The listing builds one solid part. Answer for the finished solid, in the listing's coordinates (mm). Face numbers are marked on the shaded views. A direction names the side the tool comes from. Round coordinates to 2 decimals unless told otherwise and drop trailing zeros. Loops run counter-clockwise (first coordinate to the right, second up) from the corner with the lowest first, then second, coordinate; pieces in that order, holes last. Notation, with made-up numbers: (88, 53.25) - (108, 53.25) arc R27 ccw to (108, 71.25) - close; hole circle Ø8 at (-5, -18). An arc over 180 degrees is marked (long way). Write item = value, one per line. Start each with the question number.
1) Given pin 1 Ø15 at (y, z) = (-5.5, 38) entering from -X; pin 2 Ø5 at (x, z) = (19.5, 20.5) entering from -Y; pin 3 Ø12 at (x, y) = (28.5, 0.5) entering from +Z; pin 4 Ø15 at (y, z) = (-5, 27.5) entering from +X, each flat-ended and moving along its own axis, determine where each tip first touches the part or whether it passes through.
2) Section B-B, the plane y = 17 is taken. Determine the outline of the cut face in (x, z).
3) Section C-C, the plane x = 20.5 is taken. Determine the outline of the cut face in (y, z), and give its area (3 significant figures).
4) Section D-D, the plane x = -31 is taken. Determine the outline of the cut face in (y, z).
5) A tool of negligible diameter and unlimited length cuts with its end or side. For the marked faces 4, 5, 6 and 7, from which of +Z, -Z, +X, -X, +Y, -Y can it reach the whole face along a straight path? Write none if from no direction.
6) Section A-A, the plane z = 26 is taken. Determine the outline of the cut face in (x, y).
7) For a pull along X with two mould halves and no side action, classify the marked faces 1, 2 and 3 as released by +X, released by -X, zero draft, split by the parting line, or undercut.
8) Straight lines are drawn through the part: line 1 along Y through (x, z) = (30, 6); line 2 along X through (y, z) = (17, 7); line 3 along X through (y, z) = (2.5, 22.5). For each, find the intervals that lie inside material, in ascending order.
from build123d import *

# Parameters (mm, degrees)
SKETCH_1_W          = 80
SKETCH_1_H          = 50
EXTRUDE_1_DEPTH     = 10
EXTRUDE_2_DEPTH     = 10
SKETCH_3_R          = 6
CUT_EXTRUDE_1_DEPTH = 86.732140997
SKETCH_4_R          = 4.5
CUT_EXTRUDE_2_DEPTH = 69.738635424


with BuildPart() as part:
    # 草图1 → 凸台-拉伸1 (new body)
    with BuildSketch(Plane.XY):
        Rectangle(SKETCH_1_W, SKETCH_1_H)
    extrude(amount=EXTRUDE_1_DEPTH)

    # 草图2 → 凸台-拉伸2 (add)
    with BuildSketch(Plane(origin=(15, 0, 0), x_dir=(0, 0, -1), z_dir=(1, 0, 0))):
        with BuildLine():
            Line((-9.5, -15), (-35, -15))
            ThreePointArc((-35, -15), (-50, 0), (-35, 15))
            Line((-35, 15), (-9.5, 15))
            Line((-9.5, 15), (-9.5, -15))
        make_face()
    extrude_2 = extrude(amount=EXTRUDE_2_DEPTH)

    # 镜向1: 凸台-拉伸2 across plane
    add(extrude_2.mirror(Plane(origin=(0, 0, 0), x_dir=(0, 0, 1), z_dir=(1, 0, 0))))

    # 草图3 → 切除-拉伸1 (cut, through all)
    with BuildSketch(Plane(origin=(-25, 0, 0), x_dir=(0, 0, -1), z_dir=(1, 0, 0))):
        with Locations((-35, 0)):
            Circle(SKETCH_3_R)
    extrude(amount=CUT_EXTRUDE_1_DEPTH, mode=Mode.SUBTRACT)

    # 草图4 → 切除-拉伸2 (cut, through all)
    with BuildSketch(Plane.XY):
        with Locations((30, 17)):
            Circle(SKETCH_4_R)
        with Locations((30, -17)):
            Circle(SKETCH_4_R)
        with Locations((-30, 17)):
            Circle(SKETCH_4_R)
        with Locations((-30, -17)):
            Circle(SKETCH_4_R)
    extrude(amount=CUT_EXTRUDE_2_DEPTH, mode=Mode.SUBTRACT)


solid = part.part
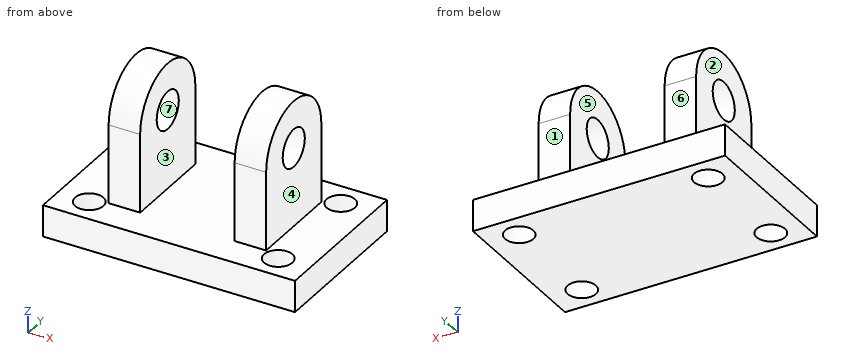
Geometry check:
q1.pin_1 = -25
q1.pin_2 = -15
q1.pin_3 = 50
q1.pin_4 = 25
q2.outline = (-40, 0) - (-34.5, 0) - (-34.5, 10) - (-40, 10) - close; (-25.5, 0) - (25.5, 0) - (25.5, 10) - (-25.5, 10) - close; (34.5, 0) - (40, 0) - (40, 10) - (34.5, 10) - close
q3.outline = (-25, 0) - (25, 0) - (25, 10) - (15, 10) - (15, 35) arc R15 ccw to (-15, 35) - (-15, 10) - (-25, 10) - close; hole circle Ø12 at (0, 35)
q3.area = 1,490 mm2
q4.outline = (-25, 0) - (-21.39, 0) - (-21.39, 10) - (-25, 10) - close; (-12.61, 0) - (12.61, 0) - (12.61, 10) - (-12.61, 10) - close; (21.39, 0) - (25, 0) - (25, 10) - (21.39, 10) - close
q5.face_4 = +Z, +X, +Y, -Y
q5.face_5 = +Z, +Y, -Y
q5.face_6 = +Z, +X, -X, +Y
q5.face_7 = +X, -X
q6.outline = (-25, -15) - (-15, -15) - (-15, 15) - (-25, 15) - close; (15, -15) - (25, -15) - (25, 15) - (15, 15) - close
q7.face_1 = zero draft
q7.face_2 = released by -X
q7.face_3 = undercut
q8.line_1 = -25 to -21.5, -12.5 to 12.5, 21.5 to 25
q8.line_2 = -40 to -34.5, -25.5 to 25.5, 34.5 to 40
q8.line_3 = -25 to -15, 15 to 25
